Input: part model. Units: mm. Frame: model coordinates. Face numbers are marked on the shaded views. A direction names the side the tool comes from. Give positions to 0.01 mm unless a question says otherwise; leave off trailing zeros. Write each loop counter-clockwise with the first axis right and the second up, starting at its lowest first coordinate (ties: lowest second). Pieces come first, ordered by that corner, then holes. Notation, with made-up numbers: (14, 74.5) - (38, 74.5) arc R12 cw to (38, 85.5) - close; hole circle Ø11 at (32, 61.5). An arc over 180 degrees is marked (long way). Use a Markdown table: item, result. Add a question column.
1. Pin query (flat end, axial travel): pin 1 (1.5 mm diameter, centred on x = -13.5, z = 25, fed in from +Y); pin 2 (5 mm diameter, centred on x = 10, z = 35, fed in from -Y); pin 3 (5 mm diameter, centred on y = -3.5, z = 26.5, fed in from -X); pin 4 (3 mm diameter, centred on y = 1, z = 15, fed in from -X). Return the tip coordinate at first contact, or that it passes through.
2. Mould query, pull axis X, two halves, no side actions, for the marked faces 1, 2 and 3. Classes: released by +X, released by -X, zero draft, split by the parting line, or undercut.
3. Section query A-A, the plane x = -20. Return loops of the section in (y, z).
4. Material intervals for probe 1 along Z at (x, y) = (10, -7.95); probe 2 along Z at (x, y) = (-27, -6.15); probe 3 along Y at (x, z) = (15, 14), sorted ascending.
5. Set-up query: the marked faces 4, 5 and 6. Return all of +Z, -Z, +X, -X, +Y, -Y with unobstructed straight access to the full face (end or side cutting, diameter ignored); none if empty.
6. Section query C-C, the plane y = 6. Return loops of the section in (x, z), plus the area to 3 significant figures.
7. Section query B-B, the plane z = 15. Return loops of the section in (x, y).
8. Section query D-D, the plane x = 0. Return loops of the section in (y, z), plus the area to 3 significant figures.
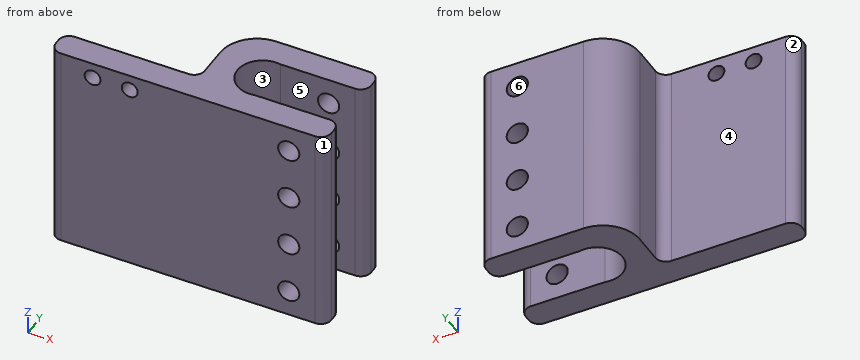
```python
from build123d import *

# Parameters (mm, degrees)
F0_W     = 25.5
F0_H     = 5
F1_DEPTH = 40
F2_R     = 2
F2_R_2   = 1.5
F3_DEPTH = 20
F4_R     = 2
F5_R     = 7


with BuildPart() as f1:
    # F0 (on Top) → F1 (new body)
    with BuildSketch(Plane.XY):
        with BuildLine():
            ThreePointArc((0.969536, -4.65), (-4.75, 0), (0.969536, 4.65))
            Line((0.969536, 4.65), (17, 4.65))
            Line((17, 4.65), (17, 9.75))
            Line((17, 9.75), (-9.5, 9.75))
            Line((-9.5, 9.75), (-9.5, -4.75))
            Line((-9.5, -4.75), (-9.5, -9.75))
            Line((-9.5, -9.75), (17, -9.75))
            Line((17, -9.75), (17, -4.65))
            Line((17, -4.65), (0.969536, -4.65))
        make_face()
        with Locations((-22.25, -7.25)):
            Rectangle(F0_W, F0_H)
    extrude(amount=F1_DEPTH)

    # F2 (on Front) → F3 (cut, symmetric)
    with BuildSketch(Plane.XZ):
        with Locations((10, 35)):
            Circle(F2_R)
        with Locations((10, 25)):
            Circle(F2_R)
        with Locations((10, 15)):
            Circle(F2_R)
        with Locations((10, 5)):
            Circle(F2_R)
        with Locations((-27, 37)):
            Circle(F2_R_2)
        with Locations((-20, 37)):
            Circle(F2_R_2)
    extrude(amount=F3_DEPTH, both=True, mode=Mode.SUBTRACT)

    # F4
    f4_edges = [f1.edges().sort_by_distance(p)[0] for p in [
        (-35, -9.75, 20),
        (-35, -4.75, 20),
        (17, -9.75, 20),
        (-9.5, -4.75, 20),
        (17, -4.65, 20),
        (17, 4.65, 20),
        (17, 9.75, 20),
    ]]
    fillet(f4_edges, radius=F4_R)

    # F5
    f5_edges = [f1.edges().sort_by_distance(p)[0] for p in [
        (-9.5, 9.75, 20),
    ]]
    fillet(f5_edges, radius=F5_R)


solid = f1.part
```
Result sheet:
| question | item | result |
|---|---|---|
| 1 | pin 1 | stops at y = -4.75 |
| 1 | pin 2 | stops at y = -9.75 |
| 1 | pin 3 | stops at x = -34.85 |
| 1 | pin 4 | stops at x = -9.5 |
| 2 | face 1 | released by +X |
| 2 | face 2 | released by -X |
| 2 | face 3 | undercut |
| 3 | outline | (-9.75, 0) - (-4.75, 0) - (-4.75, 35.5) - (-9.75, 35.5) - close; (-9.75, 38.5) - (-4.75, 38.5) - (-4.75, 40) - (-9.75, 40) - close |
| 4 | probe 1 | z = 0 to 3, 7 to 13, 17 to 23, 27 to 33, 37 to 40 |
| 4 | probe 2 | z = 0 to 35.5, 38.5 to 40 |
| 4 | probe 3 | y = -9.75 to -4.65, 4.65 to 9.75 |
| 5 | face 4 | +Z, -Z, -X, +Y |
| 5 | face 5 | +Z, -Z, +X |
| 5 | face 6 | +Y, -Y |
| 6 | outline | (-8.7, 0) - (16.89, 0) - (16.89, 40) - (-8.7, 40) - close; hole circle Ø4 at (10, 5); hole circle Ø4 at (10, 15); hole circle Ø4 at (10, 25); hole circle Ø4 at (10, 35) |
| 6 | area | 973 mm² |
| 7 | outline | (-35, -7.75) arc R2 ccw to (-33, -9.75) - (8, -9.75) - (8, -4.65) - (0.97, -4.65) arc R4.75 cw (long way) to (0.97, 4.65) - (8, 4.65) - (8, 9.75) - (-2.5, 9.75) arc R7 ccw to (-9.5, 2.75) - (-9.5, -2.75) arc R2 cw to (-11.5, -4.75) - (-33, -4.75) arc R2 ccw to (-35, -6.75) - close; (12, -9.75) - (15, -9.75) arc R2 ccw to (17, -7.75) - (17, -6.65) arc R2 ccw to (15, -4.65) - (12, -4.65) - close; (12, 4.65) - (15, 4.65) arc R2 ccw to (17, 6.65) - (17, 7.75) arc R2 ccw to (15, 9.75) - (12, 9.75) - close |
| 8 | outline | (-9.75, 0) - (-4.75, 0) - (-4.75, 40) - (-9.75, 40) - close; (4.75, 0) - (9.75, 0) - (9.75, 40) - (4.75, 40) - close |
| 8 | area | 400 mm² |
